Source: CAD feature listing. Evaluate the final solid. Frame: model axes, mm. A direction names the side the tool comes from. Give positions to 0.01 mm unless a question says otherwise; leave off trailing zeros. Order: outer loops, then holes, each group sorted by start corner. A loop starts at its lowest first (then second) coordinate and runs counter-clockwise, first axis right, second up. Notation, with made-up numbers: (-16.75, -32) -> (12.25, -32) arc R6 cw to (12.25, -26) -> close; hole circle Ø5 at (37.5, -15). An arc over 180 degrees is marked (long way). Answer in a Markdown table with one row per item.
```python
from build123d import *

# Parameters (mm, degrees)
SKETCH006_R            = 2.5
SKETCH006_R_2          = 38.75
PAD004_DEPTH           = 1.5
SKETCH007_W            = 1.5
SKETCH007_H            = 80
PAD005_DEPTH           = 1.5
LINEARPATTERN002_COUNT = 5
LINEARPATTERN002_PITCH = 15
SKETCH008_W            = 80
SKETCH008_H            = 1.5
PAD006_DEPTH           = 1.5
LINEARPATTERN003_COUNT = 5
LINEARPATTERN003_PITCH = 15
PAD007_DEPTH           = 3
SKETCH033_R            = 3.646447
SKETCH033_R_2          = 2.5
PAD017_DEPTH           = 3


with BuildPart() as part:
    # Sketch006 → Pad004 (new body)
    with BuildSketch(Plane.XY):
        with BuildLine():
            Line((40, -36), (40, 36))
            ThreePointArc((40, 36), (38.828427, 38.828427), (36, 40))
            Line((36, 40), (-36, 40))
            ThreePointArc((-36, 40), (-38.828427, 38.828427), (-40, 36))
            Line((-40, 36), (-40, -36))
            ThreePointArc((-40, -36), (-38.828427, -38.828427), (-36, -40))
            Line((-36, -40), (36, -40))
            ThreePointArc((36, -40), (38.828427, -38.828427), (40, -36))
        make_face()
        with Locations((-35.75, 35.75)):
            Circle(SKETCH006_R, mode=Mode.SUBTRACT)
        with Locations((35.75, 35.75)):
            Circle(SKETCH006_R, mode=Mode.SUBTRACT)
        with Locations((35.75, -35.75)):
            Circle(SKETCH006_R, mode=Mode.SUBTRACT)
        with Locations((-35.75, -35.75)):
            Circle(SKETCH006_R, mode=Mode.SUBTRACT)
        Circle(SKETCH006_R_2, mode=Mode.SUBTRACT)
    extrude(amount=PAD004_DEPTH)

    # Sketch007 → Pad005 (join)
    with BuildSketch(Plane.XY):
        with Locations((-30, 0)):
            Rectangle(SKETCH007_W, SKETCH007_H)
    pad005 = extrude(amount=PAD005_DEPTH)

    # LinearPattern002: Pad005 ×5
    with Locations(*[(i * LINEARPATTERN002_PITCH, 0, 0) for i in range(1, LINEARPATTERN002_COUNT)]):
        add(pad005)

    # Sketch008 → Pad006 (join)
    with BuildSketch(Plane.XY):
        with Locations((0, -30)):
            Rectangle(SKETCH008_W, SKETCH008_H)
    pad006 = extrude(amount=PAD006_DEPTH)

    # LinearPattern003: Pad006 ×5
    with Locations(*[(0, i * LINEARPATTERN003_PITCH, 0) for i in range(1, LINEARPATTERN003_COUNT)]):
        add(pad006)

    # Sketch009 (on Face137 of LinearPattern003) → Pad007 (join)
    with BuildSketch(Plane.XY.offset(1.5)):
        with BuildLine():
            Line((-40, 36), (-40, -36))
            ThreePointArc((-40, -36), (-38.828427, -38.828427), (-36, -40))
            Line((-36, -40), (36, -40))
            ThreePointArc((36, -40), (38.828427, -38.828427), (40, -36))
            Line((40, -36), (40, 36))
            ThreePointArc((40, 36), (38.828427, 38.828427), (36, 40))
            Line((36, 40), (-36, 40))
            ThreePointArc((-36, 40), (-38.828427, 38.828427), (-40, 36))
        make_face()
        with BuildLine():
            Line((-39, 36), (-39, -36))
            ThreePointArc((-39, -36), (-38.12132, -38.12132), (-36, -39))
            Line((-36, -39), (36, -39))
            ThreePointArc((36, -39), (38.12132, -38.12132), (39, -36))
            Line((39, -36), (39, 36))
            ThreePointArc((39, 36), (38.12132, 38.12132), (36, 39))
            Line((36, 39), (-36, 39))
            ThreePointArc((-36, 39), (-38.12132, 38.12132), (-39, 36))
        make_face(mode=Mode.SUBTRACT)
    extrude(amount=PAD007_DEPTH)

    # Sketch033 (on Face130 of Pad007) → Pad017 (join)
    with BuildSketch(Plane.XY.offset(1.5)):
        with Locations((35.75, 35.75)):
            Circle(SKETCH033_R)
        with Locations((35.75, 35.75)):
            Circle(SKETCH033_R_2, mode=Mode.SUBTRACT)
        with Locations((-35.75, 35.75)):
            Circle(SKETCH033_R)
        with Locations((-35.75, 35.75)):
            Circle(SKETCH033_R_2, mode=Mode.SUBTRACT)
        with Locations((-35.75, -35.75)):
            Circle(SKETCH033_R)
        with Locations((-35.75, -35.75)):
            Circle(SKETCH033_R_2, mode=Mode.SUBTRACT)
        with Locations((35.75, -35.75)):
            Circle(SKETCH033_R)
        with Locations((35.75, -35.75)):
            Circle(SKETCH033_R_2, mode=Mode.SUBTRACT)
    extrude(amount=PAD017_DEPTH)


solid = part.part
```
(1) Ray query, probe 1 along Y at (x, z) = (-24.5, 0.9); probe 2 along Y at (x, z) = (35.75, 3.4); probe 3 along Y at (x, z) = (-16, 2.3). Return the intervals inside material, ascending.
A:
| item | result |
|---|---|
| probe 1 | y = -40 to -29.25, -15.75 to -14.25, -0.75 to 0.75, 14.25 to 15.75, 29.25 to 40 |
| probe 2 | y = -40 to -38.25, -33.25 to -32.1, 32.1 to 33.25, 38.25 to 40 |
| probe 3 | y = -40 to -39, 39 to 40 |
(2) Access query for faces 1 (the flat face through (-0.6, 0.6, 0)), 2 (the cylindrical face through (-27.4, 27.4, 0.7)), 3 (the flat face through (0, -39, 3)). Directions: +Z, -Z, +X, -X, +Y, -Y. A direction counts if a zero-diameter tool reaches every point of the face in a straight line with its end or side. Return the directions, or none.
A:
| item | result |
|---|---|
| face 1 | -Z, +X, -X, +Y, -Y |
| face 2 | +Z, -Z |
| face 3 | +Z |
(3) First-contact query: pin 1 Ø1 at (x, y) = (-19, -17.5) entering from -Z. Flat tip, straight axial feed; report the tip coordinate or a pass-through.
A:
| item | result |
|---|---|
| pin 1 | passes through |
(4) Pull-direction query (Y, two-part tool) for faces 4 (the cylindrical face through (37.974, -7.716, 0.74)), 5 (the flat face through (32.4, 35.7, 4.5)), 6 (the cylindrical face through (-38.859, -38.797, 2.218)); classes: +Y half, -Y half, draft (parallel to the pull), parting line (faces both ways), or undercut.
A:
| item | result |
|---|---|
| face 4 | undercut |
| face 5 | draft |
| face 6 | -Y half |
(5) Section query A-A (x = 11). Give the number of separate pieces and of enclosed holes in the cut face, plus the area to 3 significant figures.
A:
| item | result |
|---|---|
| separate pieces | 7 |
| enclosed holes | 0 |
| area | 25.8 mm^2 |
(6) Section query C-C (z = 3.8). Return the cut outline in (x, y), plus the area to 3 significant figures.
A:
| item | result |
|---|---|
| outline | (-40, -36) arc R4 ccw to (-36, -40) -> (36, -40) arc R4 ccw to (40, -36) -> (40, 36) arc R4 ccw to (36, 40) -> (-36, 40) arc R4 ccw to (-40, 36) -> close; hole (-39, -34.1) arc R3.65 cw (long way) to (-34.1, -39) -> (34.1, -39) arc R3.65 cw (long way) to (39, -34.1) -> (39, 34.1) arc R3.65 cw (long way) to (34.1, 39) -> (-34.1, 39) arc R3.65 cw (long way) to (-39, 34.1) -> close; hole circle Ø5 at (-35.75, -35.75); hole circle Ø5 at (-35.75, 35.75); hole circle Ø5 at (35.75, -35.75); hole circle Ø5 at (35.75, 35.75) |
| area | 388 mm^2 |
